Autodesk Fusion 360 part; units mm, degrees
sketch "Sketch1" plane through (0, 0, 0) normal (0, 0, 1) x (1, 0, 0)
  line L0 (-20, 20) -> (20, 20)
  line L1 (20, 20) -> (20, -20)
  line L2 (20, -20) -> (-20, -20)
  line L3 (-20, -20) -> (-20, 20)
  line L4 (0, 0) -> (15, 0)
  line L5 (0, 0) -> (0, -12)
  line L6 (0, -12) -> (15, -12)
  line L7 (15, -12) -> (-15, -12)
  line L8 (-15, -12) -> (-15, 12)
  line L9 (-15, 12) -> (15, 12)
  line L10 (15, 12) -> (15, -12)
  circle A0 centre (-15, 12) radius 1.5
  circle A1 centre (15, 12) radius 1.5
  circle A2 centre (15, -12) radius 1.5
  circle A3 centre (-15, -12) radius 1.5
  dimension "d1" = 12
  dimension "d2" = 30
  dimension "d3" = 24
  dimension "d4" = 3
  dimension "d5" = 3
  dimension "d6" = 3
  dimension "d7" = 3
extrude "Extrude1" add sketch "Sketch1" along normal blind 12 contours L0 L1 L2 L3 | L4 L5 L7 L8 L9 L10 A0 A1 A3 | L4 L5 L6 L7 L10 A2
sketch "Sketch2" plane through (0, 0, 12) normal (0, 0, 1) x (-1, 0, 0)
  circle A0 centre (-15, -12) radius 1.5
  circle A1 centre (15, 12) radius 1.5
  circle A2 centre (15, -12) radius 1.5
  circle A3 centre (-15, 12) radius 1.5
  line L0 (20, 20) -> (-20, 20)
  line L1 (-20, 20) -> (-20, -20)
  line L2 (-20, -20) -> (20, -20)
  line L3 (20, -20) -> (20, 20)
  circle A4 centre (0, 0) radius 12.5
  dimension "d10" = 25
extrude "Extrude2" cut sketch "Sketch2" against normal blind 12 contours A4
sketch "Sketch3" plane through (0, 0, 12) normal (0, 0, 1) x (-1, 0, 0)
  circle A0 centre (0, 0) radius 12.5
  circle A1 centre (-15, -12) radius 1.5
  circle A2 centre (15, 12) radius 1.5
  circle A3 centre (15, -12) radius 1.5
  circle A4 centre (-15, 12) radius 1.5
  line L0 (20, 20) -> (-20, 20)
  line L1 (-20, 20) -> (-20, -20)
  line L2 (-20, -20) -> (20, -20)
  line L3 (20, -20) -> (20, 20)
  circle A5 centre (15, -12) radius 1.6
  circle A6 centre (-15, -12) radius 1.6
  circle A7 centre (-15, 12) radius 1.6
  circle A8 centre (15, 12) radius 1.6
  dimension "d13" = 3.2
  dimension "d14" = 3.2
  dimension "d15" = 3.2
  dimension "d16" = 3.2
extrude "Extrude3" cut sketch "Sketch3" against normal blind 12 contours A5 | A6 | A7 | A8
sketch "Sketch4" plane through (0, 0, 12) normal (0, 0, 1) x (-1, 0, 0)
  circle A0 centre (15, 12) radius 1.6
  circle A1 centre (-15, 12) radius 1.6
  circle A2 centre (15, -12) radius 1.6
  circle A3 centre (-15, -12) radius 1.6
  circle A4 centre (0, 0) radius 12.5
  line L0 (20, 20) -> (-20, 20)
  line L1 (-20, 20) -> (-20, -20)
  line L2 (-20, -20) -> (20, -20)
  line L3 (20, -20) -> (20, 20)
Source: CAD feature listing. Evaluate the final solid. Frame: model axes, mm. Round coordinates to 2 decimals unless told otherwise and drop trailing zeros. Loops run counter-clockwise (first coordinate to the right, second up) from the corner with the lowest first, then second, coordinate; pieces in that order, holes last. Notation, with made-up numbers: M 83,1.5 L 139,1.5 A36 cw 139,39.5 Z; hole C 52.25,21.5 d1. An arc over 180 degrees is marked long. Use a Markdown table: item, result. Add a question column.
1. Section query D-D on x = -15. Return the cut outline in (y, z), then the cut area to 3 significant figures.
2. Mould query, pull axis Y, two halves, no side actions, for faces 1 (the flat face through (0, 20, 6)), 2 (the cylindrical face through (-13.4, 11.93, 6.08)), 3 (the cylindrical face through (16.18, -13.08, 6.08)), 4 (the flat face through (-20, 0, 6)). Classes: pulls with the +Y half, pulls with the -Y half, needs draft (parallel to the pull), parting line crosses it, or undercut.
3. Section query A-A on x = 0. Return the cut outline in (y, z), then the cut area to 3 significant figures.
4. Section query B-B on y = 12. Return the cut outline in (x, z).
5. Line query: line 1 (Y direction, x = -15, z = 8.5); line 2 (X direction, y = 11, z = 8.75); line 3 (Y direction, x = 14, z = 8). Output: solid intervals per line, ascending.
6. Section query C-C on z = 1. Return the cut outline in (x, y).
Reported:
| question | item | result |
|---|---|---|
| 1 | outline | M -20,0 L -13.6,0 L -13.6,12 L -20,12 Z; M -10.4,0 L 10.4,0 L 10.4,12 L -10.4,12 Z; M 13.6,0 L 20,0 L 20,12 L 13.6,12 Z |
| 1 | area | 403 mm² |
| 2 | face 1 | pulls with the +Y half |
| 2 | face 2 | undercut |
| 2 | face 3 | undercut |
| 2 | face 4 | needs draft |
| 3 | outline | M -20,0 L -12.5,0 L -12.5,12 L -20,12 Z; M 12.5,0 L 20,0 L 20,12 L 12.5,12 Z |
| 3 | area | 180 mm² |
| 4 | outline | M -20,0 L -16.6,0 L -16.6,12 L -20,12 Z; M -13.4,0 L -3.5,0 L -3.5,12 L -13.4,12 Z; M 3.5,0 L 13.4,0 L 13.4,12 L 3.5,12 Z; M 16.6,0 L 20,0 L 20,12 L 16.6,12 Z |
| 5 | line 1 | y = -20 to -13.6, -10.4 to 10.4, 13.6 to 20 |
| 5 | line 2 | x = -20 to -16.25, -13.75 to -5.94, 5.94 to 13.75, 16.25 to 20 |
| 5 | line 3 | y = -20 to -13.25, -10.75 to 10.75, 13.25 to 20 |
| 6 | outline | M -20,-20 L 20,-20 L 20,20 L -20,20 Z; hole C -15,-12 d3.2; hole C -15,12 d3.2; hole C 0,0 d25; hole C 15,-12 d3.2; hole C 15,12 d3.2 |
